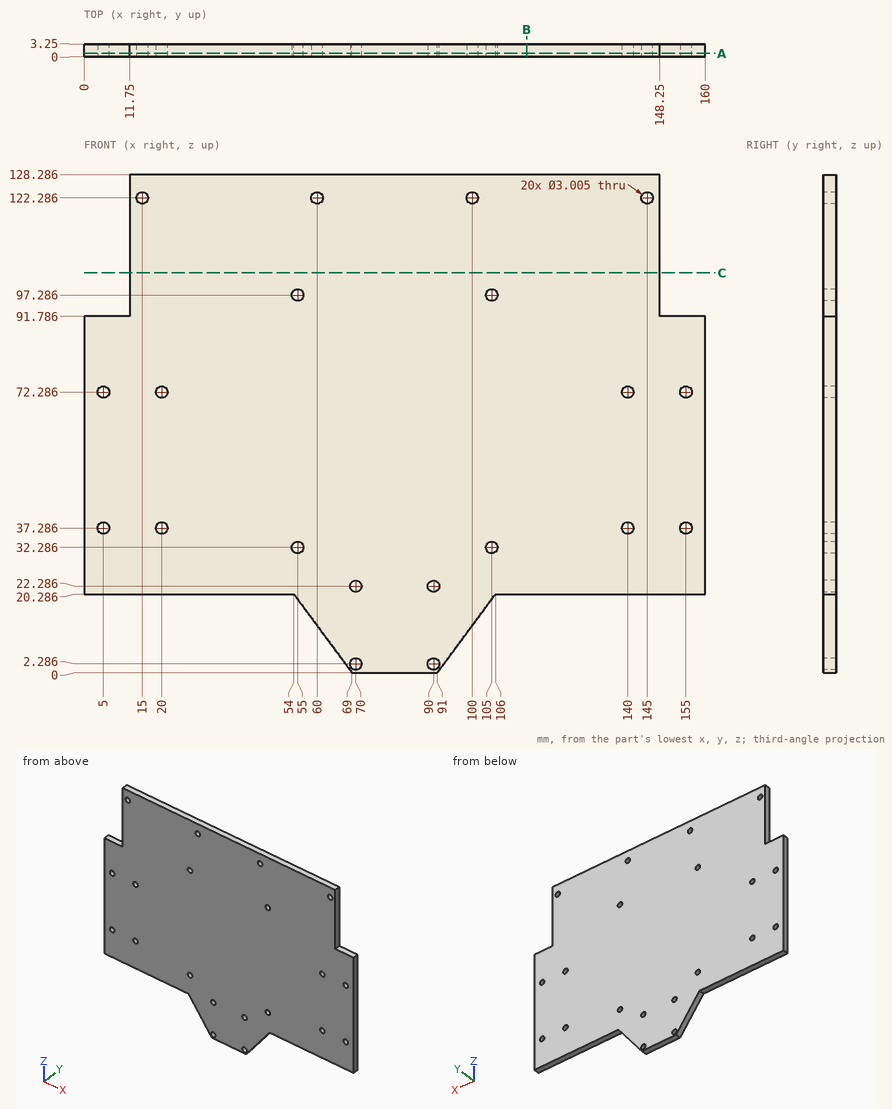
Source: three-view drawing plus pictorial views. Frame: mm from the lowest corner of the part. Round coordinates to 2 decimals unless told otherwise and drop trailing zeros. Write each loop counter-clockwise with the first axis right and the second up, starting at its lowest first coordinate (ties: lowest second). Pieces come first, ordered by that corner, then holes. Notation, with made-up numbers: M 71,58 L 99,58 A20 cw 99,97 Z; hole C 28.25,60.5 d4. An arc over 180 degrees is marked long. Write item = value, one per line.
Item 1: Section query C-C on z = 103. Return loops of the section in (x, y).
Findings:
outline = M 11.75,0 L 148.25,0 L 148.25,3.25 L 11.75,3.25 Z
Item 2: Material intervals for line 1 along X through (y, z) = (0.8, 32) (1 decimal); line 2 along X through (y, z) = (3.05, 97.5); line 3 along Z through (x, y) = (155, 1.35), sorted ascending. Write a range as [from, to].
Findings:
line_1 = [0, 53.5], [56.5, 103.5], [106.5, 160]
line_2 = [11.75, 53.51], [56.49, 103.51], [106.49, 148.25]
line_3 = [20.29, 35.78], [38.79, 70.78], [73.79, 91.79]
Item 3: Section query A-A on y = 0.85. State how many separate pieces and enclosed holes the cut face has, then the cut area to 3 significant figures.
Findings:
separate_pieces = 1
enclosed_holes = 20
area = 17,000 mm^2
Item 4: Section query B-B on x = 114. Return loops of the section in (y, z), then the cut area to 3 significant figures.
Findings:
outline = M 0,20.29 L 3.25,20.29 L 3.25,128.29 L 0,128.29 Z
area = 351 mm^2
Item 5: Pin query (flat end, axial travel): P1, Ø2.5, axis at x = 140, z = 37.29, coming from the +Y side; P2, Ø1.6, axis at y = 1.5, z = 104.5, coming from the +X side; P3, Ø1, axis at y = 2, z = 106, coming from the -X side. Return the tip coordinate at first contact, or that it passes through.
Findings:
P1 = through
P2 = 148.25
P3 = 11.75
